from build123d import *

# Parameters (mm, degrees)
ESBO_O1_W                = 150
ESBO_O1_H                = 100
RESSALTO_EXTRUS_O3_DEPTH = 6
ESBO_O3_W                = 30
ESBO_O3_H                = 6
RESSALTO_EXTRUS_O5_DEPTH = 6
ESBO_O4_W                = 6
ESBO_O4_H                = 40
RESSALTO_EXTRUS_O6_DEPTH = 6
ESBO_O5_W                = 6
ESBO_O5_H                = 40
RESSALTO_EXTRUS_O7_DEPTH = 6


with BuildPart() as part:
    # Esboço1 → Ressalto-extrusão3 (new body)
    with BuildSketch(Plane.XY):
        Rectangle(ESBO_O1_W, ESBO_O1_H)
    extrude(amount=RESSALTO_EXTRUS_O3_DEPTH)

    # Esboço3 → Ressalto-extrusão5 (add)
    with BuildSketch(Plane.XZ.offset(50)):
        with Locations((-60, 3)):
            Rectangle(ESBO_O3_W, ESBO_O3_H)
        with Locations((0, 3)):
            Rectangle(ESBO_O3_W, ESBO_O3_H)
        with Locations((60, 3)):
            Rectangle(ESBO_O3_W, ESBO_O3_H)
    extrude(amount=RESSALTO_EXTRUS_O5_DEPTH)

    # Esboço4 → Ressalto-extrusão6 (add)
    with BuildSketch(Plane(origin=(75, 0, 0), x_dir=(0, 0, -1), z_dir=(1, 0, 0))):
        with Locations((-3, 0)):
            Rectangle(ESBO_O4_W, ESBO_O4_H)
    extrude(amount=RESSALTO_EXTRUS_O6_DEPTH)

    # Esboço5 → Ressalto-extrusão7 (add)
    with BuildSketch(Plane.ZY.offset(75)):
        with Locations((3, 0)):
            Rectangle(ESBO_O5_W, ESBO_O5_H)
    extrude(amount=RESSALTO_EXTRUS_O7_DEPTH)


solid = part.part
Check sheet for the modelled part. Datum: model origin and axes. Units: mm. A direction names the side the tool comes from. Coordinates: 2 decimals unless noted, no trailing zeros. Write each loop counter-clockwise with the first axis right and the second up, starting at its lowest first coordinate (ties: lowest second). Pieces come first, ordered by that corner, then holes.
Item 1: Mould release check, pull along X, two halves, no side actions. Record for faces 1 (the face through (45, -53, 3)), 2 (the face through (75, 35, 3)), 3 (the face through (-78, 20, 3)): released by +X, released by -X, zero draft, split by the parting line, or undercut.
Numbers:
face 1: undercut
face 2: released by +X
face 3: zero draft
Item 2: Access from +Z, -Z, +X, -X, +Y, -Y to the whole of each face (thin tool, end or side, straight path). Record for faces 4 (the face through (15, -53, 3)), 5 (the face through (78, -20, 3)), 6 (the face through (78, 20, 3)), 7 (the face through (-78, -20, 3)).
Numbers:
face 4: +Z, -Z, -Y
face 5: +Z, -Z, +X, -Y
face 6: +Z, -Z, +X, +Y
face 7: +Z, -Z, -X, -Y
Item 3: Cross-section at B-B on x = 39. Record the boundary of the cut face in (y, z).
Numbers:
outline: (-50, 0) - (50, 0) - (50, 6) - (-50, 6) - close
Item 4: Cross-section at C-C on y = 36. Record the boundary of the cut face in (x, z).
Numbers:
outline: (-75, 0) - (75, 0) - (75, 6) - (-75, 6) - close
Item 5: Cross-section at A-A on z = 3.8. Record the boundary of the cut face in (x, y), then the cut area to 3 significant figures.
Numbers:
outline: (-81, -20) - (-75, -20) - (-75, -56) - (-45, -56) - (-45, -50) - (-15, -50) - (-15, -56) - (15, -56) - (15, -50) - (45, -50) - (45, -56) - (75, -56) - (75, -20) - (81, -20) - (81, 20) - (75, 20) - (75, 50) - (-75, 50) - (-75, 20) - (-81, 20) - close
area: 16,000 mm2
Item 6: Depth check by flat-ended pin: pin 1 Ø3 at (y, z) = (-53, 2.5) entering from -X; pin 2 Ø3 at (y, z) = (-53, 3.5) entering from +X; pin 3 Ø3 at (x, z) = (77.5, 2.5) entering from -Y. Enter the tip coordinate at first touch or a pass-through.
Numbers:
pin 1: stops at x = -75
pin 2: stops at x = 75
pin 3: stops at y = -20
Item 7: Scan lines: probe 1 along X at (y, z) = (-51, 2.95); probe 2 along Y at (x, z) = (26.5, 5.65); probe 3 along X at (y, z) = (44.5, 2.8). Record each from-to range of solid material in increasing order.
Numbers:
probe 1: x = -75 to -45, -15 to 15, 45 to 75
probe 2: y = -50 to 50
probe 3: x = -75 to 75
